Verification items for this drawing (mm, ordinates from the low corner). Coordinates: 2 decimals unless noted, no trailing zeros. Order: outer loops, then holes, each group sorted by start corner. A loop starts at its lowest first (then second) coordinate and runs counter-clockwise, first axis right, second up. Notation, with made-up numbers: (-39, 42) -> (0, 42) arc R29 cw to (0, 74) -> close; hole circle Ø1 at (44.25, 48). An arc over 180 degrees is marked (long way). Answer as CSV lines item,"result". Start each with the question number.
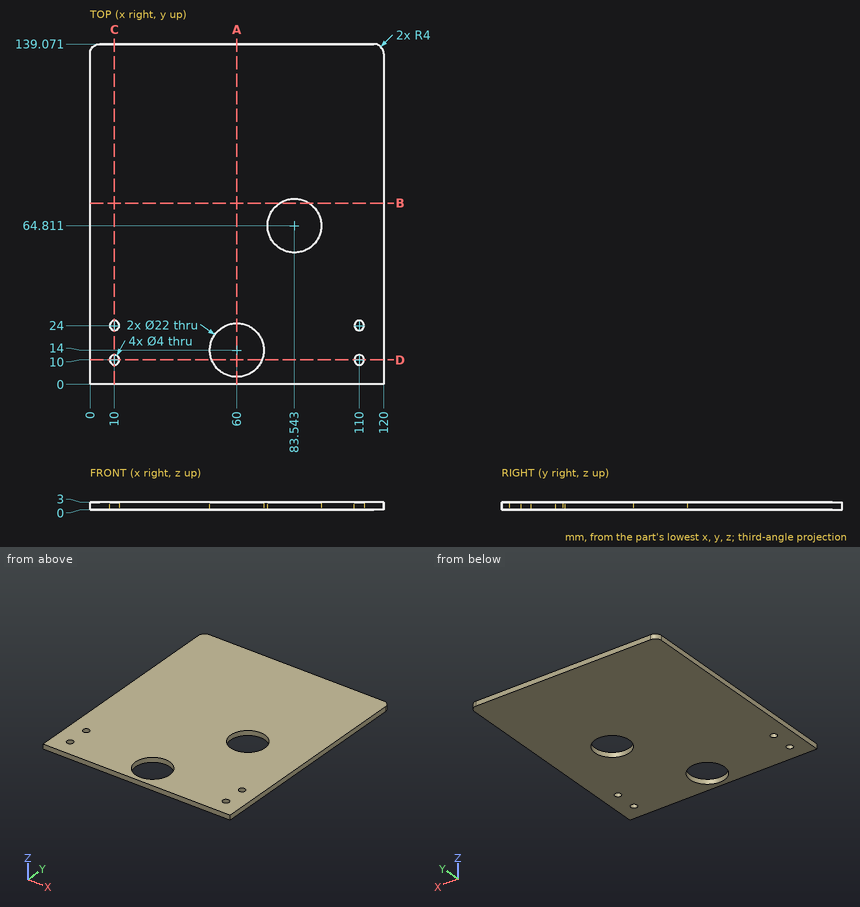
Q1. Sectioned sample at A-A, the plane x = 60. Record the cut outline in (y, z).
Q2. Thickness scan on L1, parallel to Y at x = 10, z = 2.15; L2, parallel to Y at x = 59.5, z = 0.8; L3, parallel to Y at x = 78, z = 2.85. Record the ranges inside material, lowest first.
Q3. Sectioned sample at C-C, the plane x = 10. Record the cut outline in (y, z), then the cut area to 3 significant figures.
Q4. Sectioned sample at B-B, the plane y = 74. Record the cut outline in (x, z) (1 decimal).
Q5. Sectioned sample at D-D, the plane y = 10. Record the cut outline in (x, z).
Geometry results:
1,outline,"(0, 0) -> (3, 0) -> (3, 3) -> (0, 3) -> close; (25, 0) -> (139.07, 0) -> (139.07, 3) -> (25, 3) -> close"
2,L1,"y = 0 to 8, 12 to 22, 26 to 139.07"
2,L2,"y = 0 to 3.01, 24.99 to 139.07"
2,L3,"y = 0 to 55.31, 74.31 to 139.07"
3,outline,"(0, 0) -> (8, 0) -> (8, 3) -> (0, 3) -> close; (12, 0) -> (22, 0) -> (22, 3) -> (12, 3) -> close; (26, 0) -> (139.07, 0) -> (139.07, 3) -> (26, 3) -> close"
3,area,"393 mm^2"
4,outline,"(0, 0) -> (77.5, 0) -> (77.5, 3) -> (0, 3) -> close; (89.6, 0) -> (120, 0) -> (120, 3) -> (89.6, 3) -> close"
5,outline,"(0, 0) -> (8, 0) -> (8, 3) -> (0, 3) -> close; (12, 0) -> (49.75, 0) -> (49.75, 3) -> (12, 3) -> close; (70.25, 0) -> (108, 0) -> (108, 3) -> (70.25, 3) -> close; (112, 0) -> (120, 0) -> (120, 3) -> (112, 3) -> close"
